Check sheet for the modelled part. Datum: model origin and axes. Units: mm. Face numbers are marked on the shaded views. A direction names the side the tool comes from. Round coordinates to 2 decimals unless told otherwise and drop trailing zeros. Write each loop counter-clockwise with the first axis right and the second up, starting at its lowest first coordinate (ties: lowest second). Pieces come first, ordered by that corner, then holes.
Item 1: Tool access check on the marked faces 1 and 2. Record the directions out of +Z, -Z, +X, -X, +Y, -Y that give a thin tool (end or side, any length) a straight path to the whole face; none if there is none.
Item 2: Cross-section at A-A on z = 0. Enter the section's corners in (x, y), plus the area to 3 significant figures.
Item 3: Release check for a two-part mould opening along Y. For the marked faces 3, 4 and 5 record: +Y half, -Y half, draft (parallel to the pull), parting line (faces both ways), or undercut.
Item 4: Material ranges on line 1 (Y direction, x = 3.75, z = 4.5); line 2 (Y direction, x = 2.5, z = -4.75); line 3 (X direction, y = 10.5, z = 2.75), recorded low to high.
Item 5: Cross-section at C-C on y = -18.5. Enter the section's corners in (x, z), plus the area to 3 significant figures.
Item 6: Cross-section at D-D on x = -6. Count the separate pieces of the cut face and the enclosed holes in it, plus the area to 3 significant figures.
Item 7: Cross-section at B-B on x = 0. Enter the section's corners in (y, z).
Item 8: Go/stop test with flat-tipped pins: pin 1 Ø4 at (x, y) = (-7.5, -22.5) entering from -Z; pin 2 Ø3 at (y, z) = (13.5, -6) entering from +X; pin 3 Ø4 at (y, z) = (-3.5, -3) entering from +X. Record where each tip stops, or that it passes through.
from build123d import *

# Parameters (mm, degrees)
F0_W     = 22
F0_H     = 5
F0_W_2   = 3
F2_SIZE  = 1
F3_W     = 3
F3_H     = 11.090536
F4_DEPTH = 27.256256


with BuildPart() as f1:
    # F0 (on Right) → F1 (revolve)
    with BuildSketch(Plane.YZ):
        with Locations((-11, 2.5)):
            Rectangle(F0_W, F0_H)
        Polygon((0, 5), (0, 0), (3, 0), (3, 11), (0, 9.267949), align=None)
        Polygon((-24.669873, 0), (-22, 0), (-22, 5), (-22, 7.5), (-24.669873, 7.5), align=None)
        Polygon((3, 11), (3, 0), (6, 0), (6, 5), (6, 11), align=None)
        Polygon((-29, 0), (-24.669873, 0), (-24.669873, 7.5), (-29, 5), align=None)
        with Locations((7.5, 2.5)):
            Rectangle(F0_W_2, F0_H)
        Polygon((9, 5), (9, 0), (26, 0), (26, 8), (9, 8), align=None)
    revolve(axis=Axis((0, 0.418028, 0), (0, 1, 0)))

    # F2
    f2_edges = [f1.edges().sort_by_distance(p)[0] for p in [
        (0, 9, -8),
        (0, 26, -8),
    ]]
    chamfer(f2_edges, length=F2_SIZE)

    # F3 (on Front) → F4 (cut)
    with BuildSketch(Plane.XZ):
        with Locations((11, 0)):
            Rectangle(F3_W, F3_H)
        with Locations((-11, 0)):
            Rectangle(F3_W, F3_H)
    extrude(amount=-F4_DEPTH, mode=Mode.SUBTRACT)


solid = f1.part
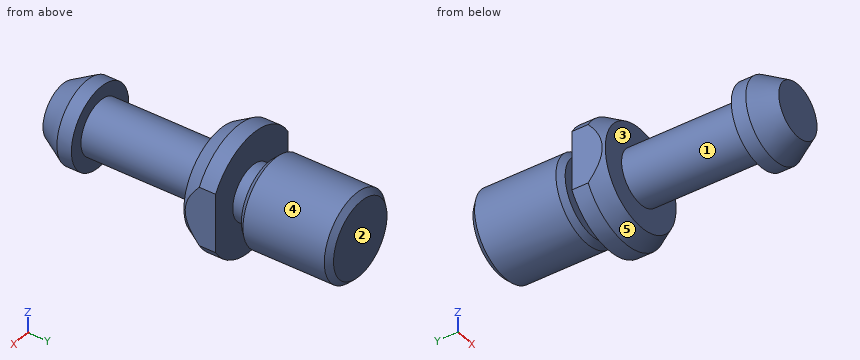
Response values:
1. face 1: none
1. face 2: +Z, -Z, +X, -X, +Y
2. outline: (-9.5, 0.4) - (-9.27, 0) - (-5, 0) - (-5, -22) - (-7.5, -22) - (-7.5, -24.67) - (-5, -29) - (5, -29) - (7.5, -24.67) - (7.5, -22) - (5, -22) - (5, 0) - (9.27, 0) - (9.5, 0.4) - (9.5, 6) - (5, 6) - (5, 9) - (7, 9) - (8, 10) - (8, 25) - (7, 26) - (-7, 26) - (-8, 25) - (-8, 10) - (-7, 9) - (-5, 9) - (-5, 6) - (-9.5, 6) - close
2. area: 728 mm2
3. face 3: undercut
3. face 4: draft
3. face 5: -Y half
4. line 1: y = -27.51 to -22, 0 to 6, 9 to 26
4. line 2: y = -28.36 to -22, 0 to 6, 9 to 26
4. line 3: x = -7.51 to 7.51
5. outline: circle Ø10 at (0, 0)
5. area: 78.5 mm2
6. separate pieces: 3
6. enclosed holes: 0
6. area: 320 mm2
7. outline: (-29, -5) - (-24.67, -7.5) - (-22, -7.5) - (-22, -5) - (0, -5) - (0, -9.27) - (3, -11) - (6, -11) - (6, -5) - (9, -5) - (9, -7) - (10, -8) - (25, -8) - (26, -7) - (26, 7) - (25, 8) - (10, 8) - (9, 7) - (9, 5) - (6, 5) - (6, 11) - (3, 11) - (0, 9.27) - (0, 5) - (-22, 5) - (-22, 7.5) - (-24.67, 7.5) - (-29, 5) - close
8. pin 1: stops at z = -5.1
8. pin 2: stops at x = 6.61
8. pin 3: stops at x = 4.9
